Here's how the part is built. I have some questions about the finished solid (model axes, mm). Face numbers are marked on the shaded views. A direction names the side the tool comes from. Give positions to 0.01 mm unless a question says otherwise; leave off trailing zeros. Loops run counter-clockwise (first coordinate to the right, second up) from the corner with the lowest first, then second, coordinate; pieces in that order, holes last. Notation, with made-up numbers: (32, -10) - (87, -10) arc R23 cw to (87, 20) - close; hole circle Ø4 at (65.5, 86.5). An arc over 180 degrees is marked (long way). Put each result on its own line as item: value. Start each with the question number.
from build123d import *

# Parameters (mm, degrees)
F0_R     = 10
F1_DEPTH = 2
F3_DEPTH = 8
F4_DEPTH = 1


with BuildPart() as f1:
    # F0 (on Top) → F1 (new body)
    with BuildSketch(Plane.XY):
        with Locations((0.104472, 0)):
            Circle(F0_R)
    extrude(amount=F1_DEPTH)

    # F2 (on face) → F3 (join)
    with BuildSketch(Plane.XY.offset(2)):
        with BuildLine():
            Line((0.7, -0.7), (0.7, -9.263617))
            ThreePointArc((0.7, -9.263617), (6.502526, -6.532934), (9.16764, -0.7))
            Line((9.16764, -0.7), (0.7, -0.7))
        make_face()
        with BuildLine():
            Line((-0.7, 0.7), (-0.7, 9.263617))
            ThreePointArc((-0.7, 9.263617), (-6.502526, 6.532934), (-9.16764, 0.7))
            Line((-9.16764, 0.7), (-0.7, 0.7))
        make_face()
    extrude(amount=F3_DEPTH)

    # F2 (on face) → F4 (cut)
    with BuildSketch(Plane.XY.offset(2)):
        with BuildLine():
            Line((0.71, 0.71), (9.367301, 0.71))
            ThreePointArc((9.367301, 0.71), (6.636361, 6.605947), (0.71, 9.270245))
            Line((0.71, 9.270245), (0.71, 0.71))
        make_face()
        with BuildLine():
            Line((-0.71, -0.71), (-9.367301, -0.71))
            ThreePointArc((-9.367301, -0.71), (-6.636361, -6.605947), (-0.71, -9.270245))
            Line((-0.71, -9.270245), (-0.71, -0.71))
        make_face()
    extrude(amount=-F4_DEPTH, mode=Mode.SUBTRACT)


solid = f1.part
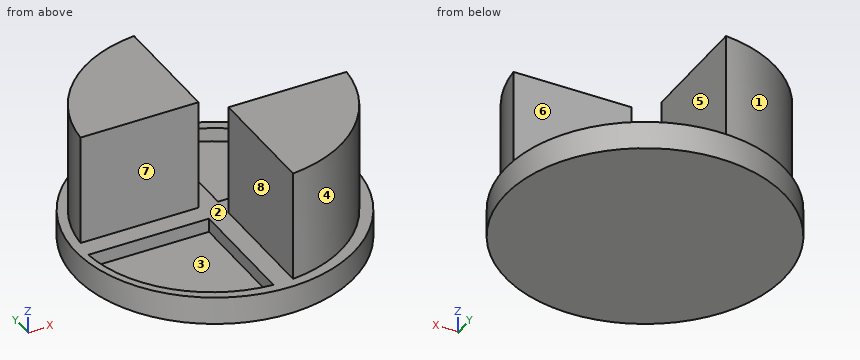
1) I'm going to push flat-ended pins straight in: P1, Ø3, axis at x = 1.5, y = 7.5, coming from the +Z side; P2, Ø2, axis at y = -4.5, z = 5, coming from the -X side; P3, Ø1.5, axis at x = 2.5, z = 1, coming from the -Y side. Where does each tip first touch, or does it pass through?
2) I need wall thicknesses on line 1 (Z direction, x = -8.5, y = -2.25); line 2 (Z direction, x = 0.5, y = -5); line 3 (X direction, y = -4, z = 8.5). Which ranges of each line are inside material? Lowest first, please.
3) Suppose I cut it at C-C on y = 3.5. Please give me the cut outline in (x, z).
4) Suppose I cut it at D-D on x = -3. Please give me the cut outline in (y, z), plus the area to 3 significant figures.
5) Suppose I cut it at B-B on z = 3.25. Please give me the cut outline in (x, y).
6) Suppose I cut it at A-A on z = 1.5. Please give me the cut outline in (x, y), plus the area to 3 significant figures.
7) Thinking about a two-plate mould opening in Y: for the marked faces 1, 2 and 3, which applies, pulls with the +Y half, pulls with the -Y half, needs draft (parallel to the pull), parting line crosses it, or undercut?
8) Which directions (+Z, -Z, +X, -X, +Y, -Y) give clear straight access to the entire face, cutting with the end or side of a thin tool? Please do the marked faces 4, 5, 6, 7 and 8.
Ans:
1. P1: stops at z = 2
1. P2: stops at x = 0.7
1. P3: stops at y = -9.86
2. line 1: z = 0 to 1
2. line 2: z = 0 to 2
2. line 3: x = 0.7 to 8.28
3. outline: (-9.26, 0) - (9.47, 0) - (9.47, 2) - (8.71, 2) - (8.71, 1) - (0.71, 1) - (0.71, 2) - (-0.7, 2) - (-0.7, 10) - (-8.51, 10) - (-8.51, 2) - (-9.26, 2) - close
4. outline: (-9.51, 0) - (9.51, 0) - (9.51, 2) - (8.76, 2) - (8.76, 10) - (0.7, 10) - (0.7, 2) - (-0.71, 2) - (-0.71, 1) - (-8.83, 1) - (-8.83, 2) - (-9.51, 2) - close
4. area: 94.4 mm²
5. outline: (-9.17, 0.7) - (-0.7, 0.7) - (-0.7, 9.26) arc R9.32 ccw to start; (0.7, -9.26) arc R9.32 ccw to (9.17, -0.7) - (0.7, -0.7) - close
6. outline: circle Ø20 at (0.1, 0); hole (-9.37, -0.71) arc R9.29 ccw to (-0.71, -9.27) - (-0.71, -0.71) - close; hole (0.71, 0.71) - (9.37, 0.71) arc R9.29 ccw to (0.71, 9.27) - close
6. area: 202 mm²
7. face 1: pulls with the +Y half
7. face 2: needs draft
7. face 3: undercut
8. face 4: +Z, +X, -Y
8. face 5: +Z, +X, +Y, -Y
8. face 6: +Z, +X, -X, +Y
8. face 7: +Z, +X, -X, -Y
8. face 8: +Z, -X, +Y, -Y
